The figure shows three views and two pictorial views of one solid part (mm, origin at its lowest corner). Answer the questions. A direction names the side the tool comes from. Coordinates: 2 decimals unless noted, no trailing zeros. Loops run counter-clockwise (first coordinate to the right, second up) from the corner with the lowest first, then second, coordinate; pieces in that order, holes last. Notation, with made-up numbers: M 89,54.5 L 141,54.5 A19 cw 141,90.5 Z; hole C -2.5,30 d5. An arc over 180 degrees is marked long. One line per item, written item: value. Start each with the question number.
1. The part is cut by section B-B (y = 19.05). Write down the section's boundary in (x, z), then the cut area to 3 significant figures.
2. The part is cut by section A-A (x = 127). Write down the section's boundary in (y, z).
3. For the marked faces 1, 2 and 3, determine the directions among +Z, -Z, +X, -X, +Y, -Y from which every point of the face is accessible in a straight line to the end or side of a thin tool.
4. The part is cut by section C-C (x = 76.5). Write down the section's boundary in (y, z), then the cut area to 3 significant figures.
5. The part is cut by section D-D (z = 24). Write down the section's boundary in (x, y).
6. Consider probe 1 along X at (y, z) = (19, 45); probe 2 along Z at (x, y) = (62, 66); probe 3 along Y at (x, z) = (17, 32.5). Determine where each line is inside the solid, lowest interval first.
7. Flat-ended cylindrical pins translate along their axes: pin 1 (11.5 mm diameter, centred on x = 90, z = 18.5, fed in from -Y); pin 2 (10 mm diameter, centred on x = 17.5, z = 24.5, fed in from +Y); pin 3 (21 mm diameter, centred on x = 79, y = 63, fed in from +Z). Find the tip coordinate at first contact, or state that the pin passes through.
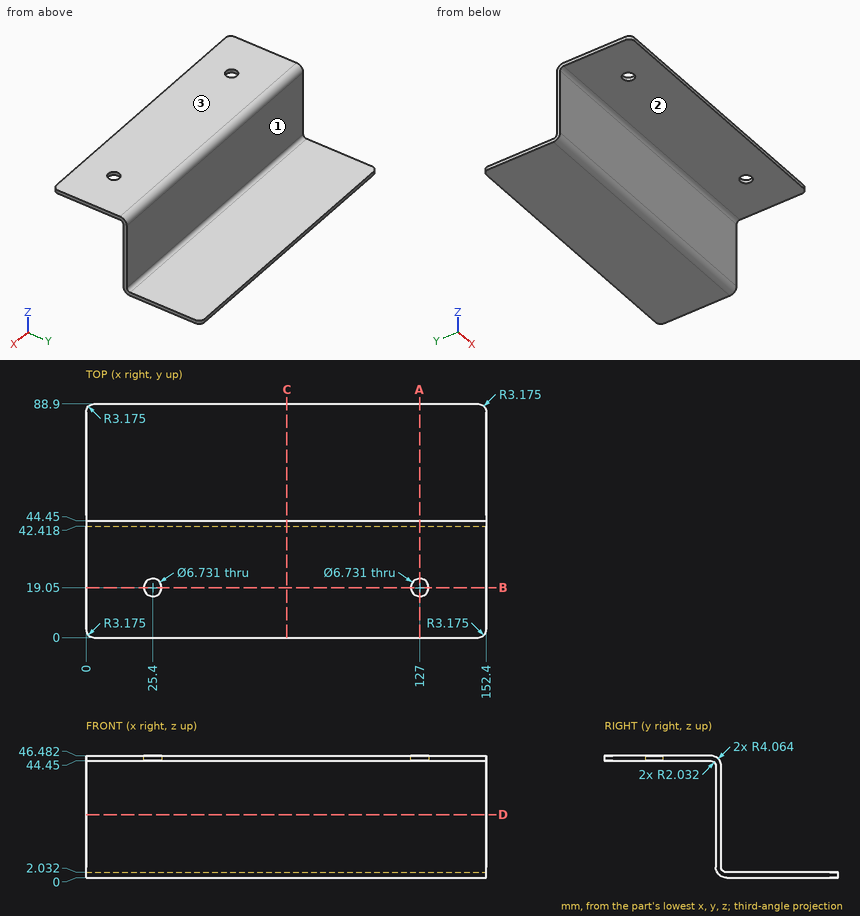
Answer block:
1. outline: M 0,44.45 L 22.03,44.45 L 22.03,46.48 L 0,46.48 Z; M 28.77,44.45 L 123.63,44.45 L 123.63,46.48 L 28.77,46.48 Z; M 130.37,44.45 L 152.4,44.45 L 152.4,46.48 L 130.37,46.48 Z
1. area: 282 mm2
2. outline: M 0,44.45 L 15.68,44.45 L 15.68,46.48 L 0,46.48 Z; M 22.42,44.45 L 40.39,44.45 A2.03 cw 42.42,42.42 L 42.42,4.06 A4.06 ccw 46.48,0 L 88.9,0 L 88.9,2.03 L 46.48,2.03 A2.03 cw 44.45,4.06 L 44.45,42.42 A4.06 ccw 40.39,46.48 L 22.42,46.48 Z
3. face 1: +Z, +X, -X, +Y
3. face 2: -Z, +X, -X, -Y
3. face 3: +Z, +X, -X, +Y, -Y
4. outline: M 0,44.45 L 40.39,44.45 A2.03 cw 42.42,42.42 L 42.42,4.06 A4.06 ccw 46.48,0 L 88.9,0 L 88.9,2.03 L 46.48,2.03 A2.03 cw 44.45,4.06 L 44.45,42.42 A4.06 ccw 40.39,46.48 L 0,46.48 Z
4. area: 266 mm2
5. outline: M 0,42.42 L 152.4,42.42 L 152.4,44.45 L 0,44.45 Z
6. probe 1: x = 0 to 22.03, 28.77 to 123.63, 130.37 to 152.4
6. probe 2: z = 0 to 2.03
6. probe 3: y = 42.42 to 44.45
7. pin 1: stops at y = 42.42
7. pin 2: stops at y = 44.45
7. pin 3: stops at z = 2.03
